```python
from build123d import *

# Parameters (mm, degrees)
SKETCH_2_R               = 4
EXTRUDE_1_DEPTH          = 15
CUT_EXTRUDE_1_DEPTH      = 38.121422387
CUT_EXTRUDE_1_DEPTH_BACK = 38.121422387
SKETCH_3_W               = 20
SKETCH_3_H               = 28
EXTRUDE_2_DEPTH          = 40


with BuildPart() as part:
    # 草图2 → 凸台-拉伸1 (new, symmetric)
    with BuildSketch(Plane(origin=(0, 0, 0), x_dir=(0, 0, -1), z_dir=(1, 0, 0))):
        with BuildLine():
            Line((-25, -8), (0, -8))
            Line((0, -8), (0, 8))
            Line((0, 8), (-25, 8))
            ThreePointArc((-25, 8), (-33, 0), (-25, -8))
        make_face()
        with Locations((-25, 0)):
            Circle(SKETCH_2_R, mode=Mode.SUBTRACT)
    extrude(amount=EXTRUDE_1_DEPTH, both=True)

    # 草图3 → 切除-拉伸1 (cut, two sides: drawn at the far end of the back side and taken through both)
    with BuildSketch(Plane(origin=(0, 0, 0), x_dir=(1, 0, 0), z_dir=(0, 1, 0)).offset(-CUT_EXTRUDE_1_DEPTH_BACK)):
        with Locations((0, -19)):
            Rectangle(SKETCH_3_W, SKETCH_3_H)
    extrude(amount=CUT_EXTRUDE_1_DEPTH + CUT_EXTRUDE_1_DEPTH_BACK, mode=Mode.SUBTRACT)

    # 草图4 → 凸台-拉伸2 (add)
    with BuildSketch(Plane(origin=(0, 0, 0), x_dir=(-1, 0, 0), z_dir=(0, 0, -1))):
        with BuildLine():
            Line((-3, -4), (3, -4))
            ThreePointArc((3, -4), (5, 0), (3, 4))
            Line((3, 4), (-3, 4))
            ThreePointArc((-3, 4), (-5, 0), (-3, -4))
        make_face()
    extrude(amount=EXTRUDE_2_DEPTH)


solid = part.part
```
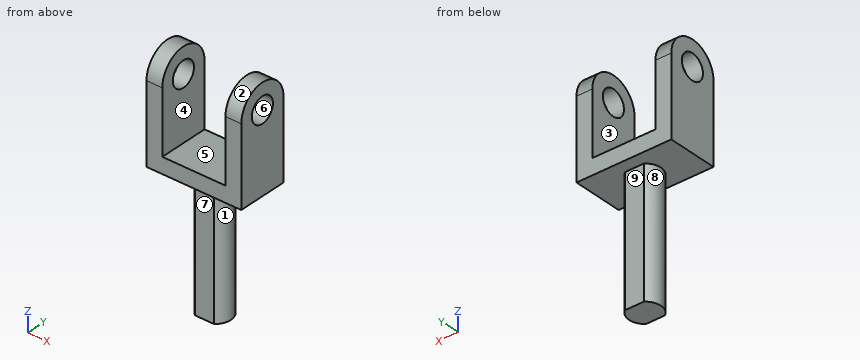
Work out the finished part from the listing and answer in its coordinate system (mm). Face numbers are marked on the shaded views. A direction names the side the tool comes from. Give positions to 0.01 mm unless a question says otherwise; leave off trailing zeros. Loops run counter-clockwise (first coordinate to the right, second up) from the corner with the lowest first, then second, coordinate; pieces in that order, holes last. Notation, with made-up numbers: (49.5, 86) -> (97.5, 86) arc R33 ccw to (97.5, 115) -> close; hole circle Ø9 at (-19, 13.25). An arc over 180 degrees is marked (long way). One line per question, with ' | ' between items. Start each with the question number.
1) Straight lines are drawn through the part: L1, parallel to Z at x = 13.95, y = 0; L2, parallel to Y at x = 11.8, z = 25; L3, parallel to X at y = -6, z = 24. For each, find the intervals that lie inside material, in ascending order.
2) Section A-A, the plane y = 0 is taken. Determine the outline of the cut face in (x, z), then the cut area to 3 significant figures.
3) Section C-C, the plane z = 23.5 is taken. Determine the outline of the cut face in (x, y).
4) Each of these flat-tipped pins is pushed along its axis until it touches: pin 1 (5 mm diameter, centred on x = 3, y = -2, fed in from +Z); pin 2 (8 mm diameter, centred on y = -3.5, z = 24, fed in from +X); pin 3 (4 mm diameter, centred on x = 5.5, z = -31.5, fed in from +Y); pin 4 (2 mm diameter, centred on x = 5.5, z = -27.5, fed in from -Y). Where does it stop, or does it pass through?
5) Section D-D, the plane y = -6.5 is taken. Determine the outline of the cut face in (x, z), then the cut area to 3 significant figures.
6) For the marked faces 5, 6, 7, 8 and 9, determine the directions among +Z, -Z, +X, -X, +Y, -Y from which every point of the face is accessible in a straight line to the end or side of a thin tool.
7) Determine the mould class of the marked faces 1, 2, 3 and 4 for opening direction X: +X half, -X half, draft (parallel to the pull), parting line (faces both ways), or undercut.
8) Section B-B, the plane x = 2 is taken. Determine the outline of the cut face in (y, z), then the cut area to 3 significant figures.
Resolved:
1) L1: 0 to 21, 29 to 33 | L2: -8 to -4, 4 to 8 | L3: -15 to -10, 10 to 15
2) outline: (-15, 0) -> (-5, 0) -> (-5, -40) -> (5, -40) -> (5, 0) -> (15, 0) -> (15, 21) -> (10, 21) -> (10, 5) -> (-10, 5) -> (-10, 21) -> (-15, 21) -> close; (-15, 29) -> (-10, 29) -> (-10, 33) -> (-15, 33) -> close; (10, 29) -> (15, 29) -> (15, 33) -> (10, 33) -> close | area: 750 mm2
3) outline: (-15, -8) -> (-10, -8) -> (-10, -3.71) -> (-15, -3.71) -> close; (-15, 3.71) -> (-10, 3.71) -> (-10, 8) -> (-15, 8) -> close; (10, -8) -> (15, -8) -> (15, -3.71) -> (10, -3.71) -> close; (10, 3.71) -> (15, 3.71) -> (15, 8) -> (10, 8) -> close
4) pin 1: z = 5 | pin 2: x = 15 | pin 3: y = 3.57 | pin 4: y = -2.18
5) outline: (-15, 0) -> (15, 0) -> (15, 29.66) -> (10, 29.66) -> (10, 5) -> (-10, 5) -> (-10, 29.66) -> (-15, 29.66) -> close | area: 397 mm2
6) face 5: +Z, +Y, -Y | face 6: +X, -X | face 7: -Z, +X, -X, -Y | face 8: -Z, -X | face 9: -Z, +X, -X, +Y
7) face 1: +X half | face 2: draft | face 3: undercut | face 4: undercut
8) outline: (-8, 0) -> (-4, 0) -> (-4, -40) -> (4, -40) -> (4, 0) -> (8, 0) -> (8, 5) -> (-8, 5) -> close | area: 400 mm2
